For this review, use the dimensioned drawing (mm, ordinates from the lowest corner) and the shaded views. A direction names the side the tool comes from. Round coordinates to 2 decimals unless told otherwise and drop trailing zeros. Loops run counter-clockwise (first coordinate to the right, second up) from the corner with the lowest first, then second, coordinate; pieces in that order, holes last. Notation, with made-up numbers: (63, -6) - (100, -6) arc R30 cw to (100, 30) - close; hole circle Ø4 at (64, -11.75). An arc over 180 degrees is marked (long way). Return JSON: item names as keys, results as strings. Group by question number.
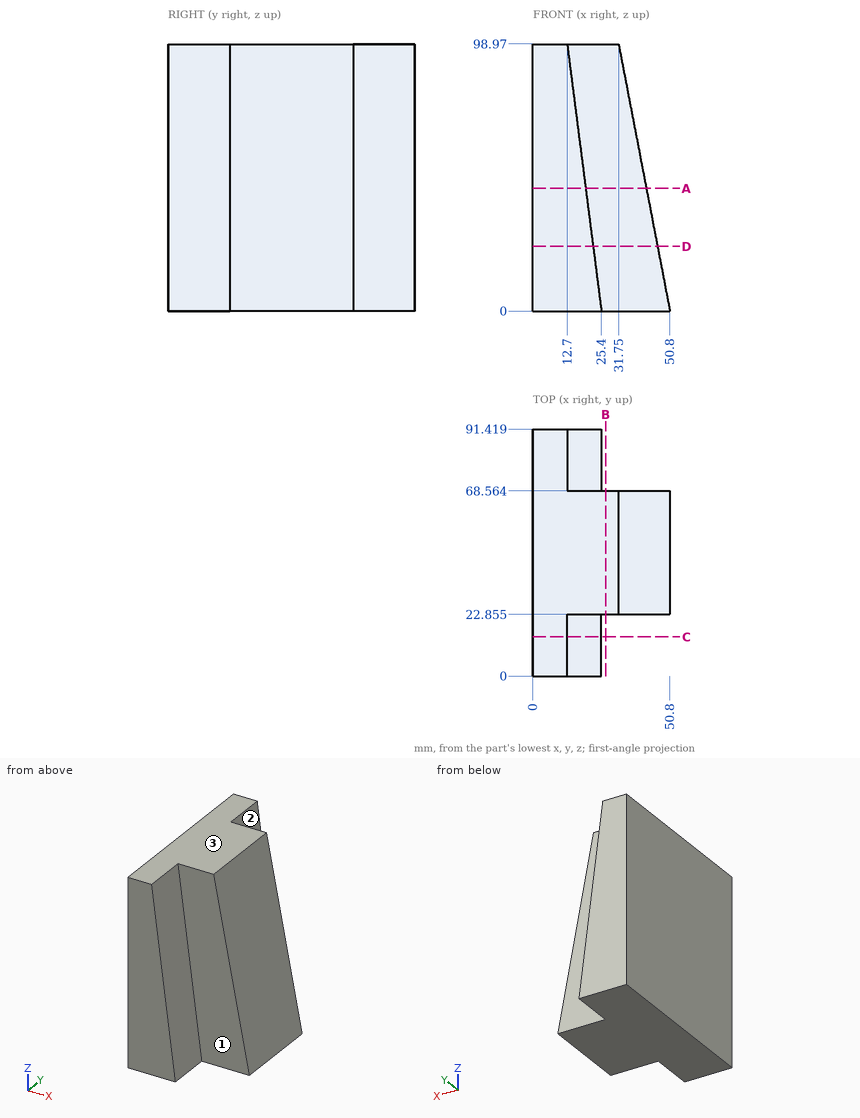
Q1. Add section A-A, the plane z = 45.5. State the section outline as (x, y) points (1 decimal), plus the area to 3 significant figures.
Q2. Add section C-C, the plane y = 14.5. State the section outline as (x, z) points, plus the area to 3 significant figures.
Q3. Add section D-D, the plane z = 24. State the section outline as (x, y) points (1 decimal).
Q4. For line 1 (Y direction, x = 46.5, z = 6) (1 decimal); line 2 (X direction, y = 30.5, z = 84.5) (1 decimal); line 3 (X direction, y = 79.5, z = 44.5), list the stretches that pass through material, from the lowest coordinate up.
Q5. Tool access review of the marked faces 1, 2 and 3: name each direction out of +Z, -Z, +X, -X, +Y, -Y from which nothing blocks a thin tool from reaching the whole face with its end or side.
Q6. Insertion check: pin 1 Ø10 at (x, z) = (27.5, 60.5) entering from -Y (1 decimal); pin 2 Ø6 at (y, z) = (17.5, 76.5) entering from +X. Each pin has a flat end and moves straight along its axis. Give the tip position at first contact, or say it passes through.
Q7. Add section B-B, the plane x = 27. State the section outline as (y, z) points (1 decimal).
Evaluation:
{
 "1": {"outline": "(0, 0) - (19.6, 0) - (19.6, 22.9) - (42, 22.9) - (42, 68.6) - (19.6, 68.6) - (19.6, 91.4) - (0, 91.4) - close", "area": "2,820 mm²"},
 "2": {"outline": "(0, 0) - (25.4, 0) - (12.7, 98.97) - (0, 98.97) - close", "area": "1,890 mm²"},
 "3": {"outline": "(0, 0) - (22.3, 0) - (22.3, 22.9) - (46.2, 22.9) - (46.2, 68.6) - (22.3, 68.6) - (22.3, 91.4) - (0, 91.4) - close"},
 "4": {"line 1": "22.9 to 68.6", "line 2": "0 to 34.5", "line 3": "0 to 19.69"},
 "5": {"face 1": "+Z, +X, -Y", "face 2": "+Z, +X, +Y", "face 3": "+Z, +X, -X, +Y, -Y"},
 "6": {"pin 1": "y = 22.9", "pin 2": "x = 15.97"},
 "7": {"outline": "(22.9, 0) - (68.6, 0) - (68.6, 99) - (22.9, 99) - close"}
}
